The model under review builds one solid part; all positions refer to its coordinate system, in mm. Face numbers are marked on the shaded views. Coordinates: 2 decimals unless noted, no trailing zeros. Use CSV: the item, a comma, the result in double quotes. Start each with the question number.
1. Clearance check with flat-ended pins moving along their axes: P1, Ø3, axis at y = -58, z = 4.5, coming from the +X side; P2, Ø12, axis at x = 10.5, y = -61.5, coming from the -Z side. State where each tip first meets the part, or that it passes through.
2. For L1, parallel to Y at x = -43.5, z = 0.5; L2, parallel to X at y = -57, z = 4.8; L3, parallel to Y at x = 0, z = 1.25, list the stretches that pass through material, from the lowest coordinate up.
3. Draft analysis for pull direction X (two halves, no side actions). For the marked faces 1 and 2, state which applies: +X half, -X half, draft (parallel to the pull), parting line (faces both ways), or undercut.
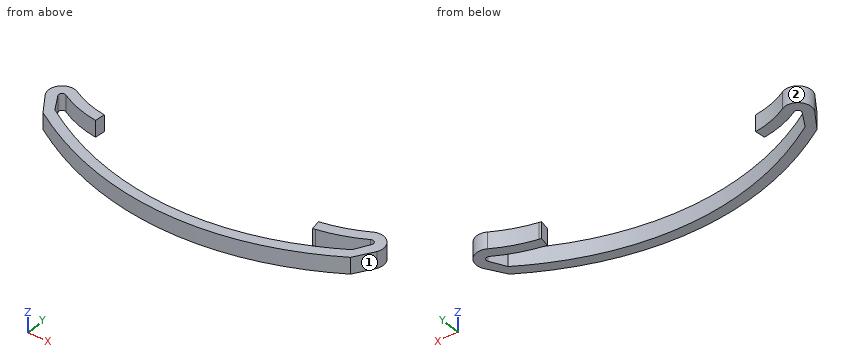
Autodesk Inventor part; units mm, degrees
ref_plane "YZ Plane" through (0, 0, 0) normal (1, 0, 0) x (0, 1, 0)
ref_plane "XZ Plane" through (0, 0, 0) normal (0, 1, 0) x (-1, 0, 0)
ref_plane "XY Plane" through (0, 0, 0) normal (0, 0, 1) x (1, 0, 0)
sketch "スケッチ1" plane through (0, 0, 0) normal (0, 0, 1) x (1, 0, 0)
  arc A0 (47.1325, -53.2266) -> (45.758, -51.8784) centre (46.2557, -52.7457) ccw
  arc A1 (33.009, -56.7784) -> (45.758, -51.8784) centre (23.6069, -13.28) ccw
  arc A2 (11.1932, -28.6204) -> (33.009, -56.7784) centre (28.8377, -37.4801) ccw
  arc A3 (11.1932, -28.6204) -> (-11.1841, -28.6384) centre (0, -23) ccw
  arc A4 (-22.0046, -54.1258) -> (-11.1841, -28.6384) centre (-27.3796, -36.8033) ccw
  arc A5 (-45.6895, -51.9306) -> (-22.0046, -54.1258) centre (-31.2017, -24.4856) ccw
  arc A6 (-45.6895, -51.9306) -> (-47.014, -53.3291) centre (-46.1563, -52.815) ccw
  line L0 (-47.014, -53.3291) -> (-44.145, -58.1151)
  spline S0 degree 4 poles (-44.145, -58.1151) (-43.8381, -58.3003) (-43.4088, -58.5568) (-42.8575, -58.8816) (-42.1841, -59.2711) (-41.6963, -59.5497) (-41.2094, -59.8243) (-40.7232, -60.0949) (-40.2377, -60.3617) (-39.7528, -60.6247) (-39.2684, -60.8839) (-38.7844, -61.1395) (-38.3007, -61.3914) (-37.8172, -61.6398) (-37.334, -61.8846) (-36.8508, -62.1259) (-36.3678, -62.3637) (-35.8847, -62.5981) (-35.4015, -62.8291) (-34.9183, -63.0567) (-34.4349, -63.281) (-33.9513, -63.502) (-33.4675, -63.7196) (-32.9834, -63.934) (-32.499, -64.1451) (-32.0143, -64.3529) (-31.5292, -64.5576) (-31.0437, -64.7589) (-30.5578, -64.9571) (-30.0715, -65.1521) (-29.5847, -65.3439) (-29.0974, -65.5325) (-28.6097, -65.7179) (-28.1214, -65.9001) (-27.6326, -66.0792) (-27.1433, -66.2551) (-26.6534, -66.4278) (-26.163, -66.5974) (-25.6721, -66.7638) (-25.1806, -66.927) (-24.6885, -67.0871) (-24.1958, -67.244) (-23.7026, -67.3978) (-23.2087, -67.5484) (-22.7144, -67.6958) (-22.2194, -67.8401) (-21.7238, -67.9811) (-21.2277, -68.1191) (-20.7311, -68.2538) (-20.2338, -68.3854) (-19.736, -68.5137) (-19.2377, -68.6389) (-18.7388, -68.7609) (-18.2393, -68.8798) (-17.7394, -68.9954) (-17.2389, -69.1078) (-16.7379, -69.217) (-16.2363, -69.323) (-15.7343, -69.4258) (-15.2318, -69.5254) (-14.7289, -69.6218) (-14.2255, -69.7149) (-13.7216, -69.8049) (-13.2173, -69.8915) (-12.7125, -69.975) (-12.2074, -70.0552) (-11.7018, -70.1322) (-11.1959, -70.2059) (-10.6896, -70.2764) (-10.1829, -70.3436) (-9.6759, -70.4075) (-9.1686, -70.4683) (-8.661, -70.5257) (-8.1531, -70.5799) (-7.6449, -70.6308) (-7.1364, -70.6784) (-6.6277, -70.7228) (-6.1188, -70.7639) (-5.6096, -70.8017) (-5.1003, -70.8362) (-4.5907, -70.8674) (-4.0811, -70.8954) (-3.5712, -70.9201) (-3.0613, -70.9415) (-2.5513, -70.9596) (-2.0411, -70.9744) (-1.5309, -70.9859) (-1.0206, -70.9941) (-0.5103, -70.9991) (0, -71.0007) (0.5103, -70.9991) (1.0206, -70.9941) (1.5309, -70.9859) (2.0411, -70.9744) (2.5512, -70.9596) (3.0613, -70.9415) (3.5712, -70.9201) (4.0811, -70.8954) (4.5907, -70.8674) (5.1002, -70.8362) (5.6096, -70.8017) (6.1187, -70.7639) (6.6276, -70.7228) (7.1363, -70.6784) (7.6447, -70.6308) (8.1529, -70.5799) (8.6608, -70.5257) (9.1683, -70.4683) (9.6756, -70.4076) (10.1825, -70.3436) (10.6891, -70.2764) (11.1953, -70.2059) (11.7011, -70.1322) (12.2065, -70.0553) (12.7115, -69.9751) (13.2161, -69.8917) (13.7202, -69.805) (14.2238, -69.7151) (14.727, -69.622) (15.2297, -69.5257) (15.7318, -69.4261) (16.2335, -69.3234) (16.7346, -69.2175) (17.2352, -69.1083) (17.7352, -68.996) (18.2346, -68.8805) (18.7335, -68.7617) (19.2317, -68.6399) (19.7293, -68.5148) (20.2264, -68.3866) (20.7227, -68.2552) (21.2185, -68.1207) (21.7136, -67.983) (22.208, -67.8421) (22.7018, -67.6981) (23.1948, -67.551) (23.6872, -67.4008) (24.1789, -67.2474) (24.6699, -67.0909) (25.1602, -66.9313) (25.6497, -66.7686) (26.1386, -66.6028) (26.6267, -66.4339) (27.1141, -66.2618) (27.6008, -66.0867) (28.0867, -65.9085) (28.5719, -65.7272) (29.0563, -65.5428) (29.54, -65.3554) (30.023, -65.1648) (30.5052, -64.9712) (30.9867, -64.7745) (31.4674, -64.5748) (31.9475, -64.3719) (32.4267, -64.166) (32.9053, -63.9571) (33.3831, -63.745) (33.8603, -63.5299) (34.3367, -63.3117) (34.8124, -63.0904) (35.2875, -62.8661) (35.7619, -62.6386) (36.2356, -62.4081) (36.7086, -62.1745) (37.181, -61.9378) (37.6528, -61.698) (38.124, -61.455) (38.5946, -61.209) (39.0646, -60.9598) (39.5341, -60.7075) (40.003, -60.452) (40.4714, -60.1934) (40.9394, -59.9316) (41.4069, -59.6666) (41.8739, -59.3984) (42.3406, -59.127) (42.8069, -58.8523) (43.4481, -58.4698) (43.9715, -58.1517) (44.3779, -57.9011) (44.6679, -57.7205) knots 0 0 0 0 0 0.014541 0.020333 0.02611 0.031872 0.03762 0.043355 0.049078 0.054789 0.060489 0.066178 0.071857 0.077527 0.083187 0.088839 0.094483 0.10012 0.105749 0.111371 0.116986 0.122595 0.128199 0.133797 0.139389 0.144976 0.150559 0.156136 0.16171 0.167279 0.172845 0.178407 0.183965 0.18952 0.195072 0.20062 0.206166 0.211709 0.21725 0.222788 0.228323 0.233857 0.239388 0.244918 0.250445 0.255971 0.261495 0.267017 0.272538 0.278057 0.283575 0.289092 0.294608 0.300122 0.305635 0.311147 0.316658 0.322169 0.327678 0.333186 0.338694 0.344201 0.349707 0.355213 0.360718 0.366222 0.371726 0.377229 0.382732 0.388235 0.393737 0.399238 0.404739 0.41024 0.415741 0.421241 0.426741 0.432241 0.43774 0.44324 0.448739 0.454238 0.459737 0.465236 0.470734 0.476233 0.481731 0.48723 0.492728 0.498227 0.503725 0.509224 0.514722 0.520221 0.525719 0.531218 0.536717 0.542216 0.547715 0.553214 0.558714 0.564214 0.569713 0.575214 0.580714 0.586215 0.591716 0.597217 0.602718 0.60822 0.613723 0.619225 0.624728 0.630232 0.635736 0.641241 0.646746 0.652251 0.657758 0.663264 0.668772 0.67428 0.679789 0.685299 0.690809 0.69632 0.701832 0.707345 0.712859 0.718374 0.72389 0.729407 0.734925 0.740444 0.745965 0.751487 0.75701 0.762535 0.768061 0.773588 0.779117 0.784648 0.790181 0.795715 0.801252 0.80679 0.812331 0.817873 0.823418 0.828965 0.834515 0.840067 0.845622 0.85118 0.85674 0.862304 0.867871 0.873441 0.879014 0.884591 0.890172 0.895757 0.901345 0.906938 0.912535 0.918137 0.923743 0.929355 0.934971 0.940593 0.946221 0.951854 0.957493 0.963139 0.968791 0.974449 0.980115 0.985788 1 1 1 1 1
  line L1 (44.6679, -57.7205) -> (47.1325, -53.2266)
  arc A7 (4.5969, -37.0887) -> (23.8174, -61.1986) centre (28.8377, -37.4801) ccw
  spline S1 degree 3 poles (23.923, -63.1268) (24.0467, -63.086) (24.1612, -63.0216) (24.3592, -62.8523) (24.4407, -62.7492) (24.5595, -62.5175) (24.5958, -62.3911) (24.6178, -62.1316) (24.6033, -62.0009) (24.5251, -61.7525) (24.4622, -61.6371) (24.3075, -61.4513) (24.2222, -61.3781) (24.0311, -61.2629) (23.9266, -61.2217) (23.8174, -61.1986) knots 0 0 0 0 0.148947 0.148947 0.297893 0.297893 0.44684 0.44684 0.595787 0.595787 0.744733 0.744733 0.872367 0.872367 1 1 1 1
  spline S2 degree 3 poles (23.923, -63.1268) (23.6264, -63.2244) (21.6991, -63.8462) (18.9298, -64.6237) (14.7719, -65.5721) (11.4157, -66.1631) (7.1944, -66.6887) (3.8013, -66.9375) (-0.4475, -67.0324) (-3.8473, -66.9351) (-8.0854, -66.5978) (-11.4616, -66.156) (-15.6527, -65.3916) (-18.978, -64.6118) (-23.0925, -63.431) (-25.7434, -62.5289) (-27.5645, -61.8359) (-27.7718, -61.756) knots -0.770978 -0.770978 -0.770978 -0.770978 -0.760435 -0.70257 -0.673637 -0.615772 -0.58684 -0.528974 -0.500042 -0.442177 -0.413244 -0.355379 -0.326446 -0.268581 -0.239649 -0.181783 -0.174342 -0.174342 -0.174342 -0.174342
  spline S3 degree 3 poles (-27.5161, -59.8282) (-27.6456, -59.8417) (-27.7712, -59.8804) (-28.0006, -60.0037) (-28.1022, -60.0872) (-28.2675, -60.2884) (-28.3298, -60.4042) (-28.4064, -60.6531) (-28.42, -60.7838) (-28.3964, -61.0432) (-28.3594, -61.1693) (-28.2435, -61.3919) (-28.1687, -61.4881) (-27.9885, -61.6491) (-27.8845, -61.7126) (-27.7718, -61.756) knots 0 0 0 0 0.145866 0.145866 0.291731 0.291731 0.437597 0.437597 0.583462 0.583462 0.729328 0.729328 0.864664 0.864664 1 1 1 1
  arc A8 (-27.5161, -59.8282) -> (-20.671, -58.4236) centre (-31.2017, -24.4856) ccw
  arc A9 (-20.671, -58.4236) -> (-4.7434, -37.0245) centre (-27.3796, -36.8033) ccw
  arc A10 (-3.4858, -36.0681) -> (-4.7434, -37.0245) centre (-3.7435, -37.0343) ccw
  arc A11 (-3.4858, -36.0681) -> (3.3494, -36.1037) centre (0, -23) ccw
  arc A12 (4.5969, -37.0887) -> (3.3494, -36.1037) centre (3.597, -37.0726) ccw
  circle A13 centre (0, -23) radius 8.525
  circle A14 centre (0, 0) radius 1.5
  circle A15 centre (-6.3066, -8.8137) radius 1.5
  line L2 (5.2372, 1.6799) -> (11.9265, -19.1744)
  arc A16 (5.2372, 1.6799) -> (-4.7491, 2.7742) centre (0, 0) ccw
  line L3 (-4.7491, 2.7742) -> (-10.1922, -6.5439)
  arc A17 (-10.1922, -6.5439) -> (-10.7715, -8.253) centre (-6.3066, -8.8137) ccw
  line L4 (-10.7715, -8.253) -> (-12.4274, -21.4394)
  arc A18 (11.9265, -19.1744) -> (-12.4274, -21.4394) centre (0, -23) ccw
  arc A19 (-9.0832, -7.6778) -> (-5.0879, -11.555) centre (-6.3066, -8.8137) ccw
  line L5 (-9.0832, -7.6778) -> (-4.9441, 2.4403)
sketch "スケッチ2" plane through (0, 0, 0) normal (0, 0, 1) x (1, 0, 0)
  spline S0 degree 4 poles (-44.145, -58.1151) (-37.6182, -62.054) (-28.2694, -66.5348) (-15.5407, -70.2705) (0.4425, -71.3509) (16.3869, -70.0942) (29.0453, -66.236) (38.314, -61.6764) (44.6679, -57.7205) knots 0 0 0 0 0 0.314296 0.438586 0.562663 0.686902 1 1 1 1 1
  arc A0 (-45.6895, -51.9306) -> (-47.014, -53.3292) centre (-46.1563, -52.815) ccw
  arc A1 (-45.6895, -51.9306) -> (-34.0657, -55.3875) centre (-31.2017, -24.4856) ccw
  arc A2 (-22.0045, -54.1258) -> (-11.1841, -28.6384) centre (-27.3796, -36.8033) ccw
  arc A3 (32.2678, -56.9238) -> (33.009, -56.7784) centre (28.8377, -37.4801) ccw
  arc A4 (33.009, -56.7784) -> (45.758, -51.8784) centre (23.6069, -13.28) ccw
  arc A5 (47.1325, -53.2266) -> (45.758, -51.8784) centre (46.2557, -52.7457) ccw
  arc A6 (-22.8936, -51.2605) -> (-13.8629, -29.9889) centre (-27.3796, -36.8033) ccw
  arc A7 (-44.289, -49.2776) -> (-33.7888, -52.4003) centre (-31.2017, -24.4856) ccw
  arc A8 (-44.289, -49.2776) -> (-49.5871, -54.8716) centre (-46.1563, -52.815) ccw
  arc A9 (31.7303, -53.9723) -> (32.3752, -53.8461) centre (28.8377, -37.4801) ccw
  arc A10 (32.3752, -53.8461) -> (44.2648, -49.2764) centre (23.6069, -13.28) ccw
  arc A11 (49.7629, -54.6691) -> (44.2648, -49.2764) centre (46.2557, -52.7457) ccw
  line L0 (-49.5871, -54.8716) -> (-45.6951, -60.6836)
  line L1 (46.2535, -60.2673) -> (49.7629, -54.6691)
  line L2 (-33.7888, -52.4003) -> (-34.0657, -55.3875)
  line L3 (-47.014, -53.3292) -> (-44.145, -58.1151)
  line L4 (44.6679, -57.7205) -> (47.1325, -53.2266)
  line L5 (31.7303, -53.9723) -> (32.2678, -56.9238)
  spline S1 degree 5 poles (-45.6951, -60.6836) (-37.3741, -65.7056) (-28.5032, -69.8262) (-19.0469, -72.6542) (0.3831, -75.4348) (19.7882, -72.4725) (29.1916, -69.5658) (38.0209, -65.3927) (46.2535, -60.2673) knots 0 0 0 0 0 0 0.500557 0.500557 0.500557 1 1 1 1 1 1
  point P0 (0, 0)
  point P1 (11.1932, -28.6204)
  point P2 (-33.3656, -63.7642)
  point P3 (-22.3576, -67.7993)
  point P4 (-11.0481, -70.226)
  point P5 (0.4419, -70.9986)
  point P6 (11.9239, -70.0979)
  point P7 (23.204, -67.5475)
  point P8 (34.1337, -63.4043)
  dimension "d0" = 3
  dimension "d1" = 3
  dimension "d2" = 3
extrude "押し出し1" add sketch "スケッチ2" along normal blind 5
properties part number "脚ゴム" material "ゴム、シリコーン"
Computed:
1,P1,"stops at x = 48.62"
1,P2,"passes through"
2,L1,"y = -61.97 to -58.5, -52.98 to -49.68"
2,L2,"x = -48.16 to -44.81, 45.06 to 48.3"
2,L3,"y = -74 to -71"
3,face 1,"+X half"
3,face 2,"undercut"
